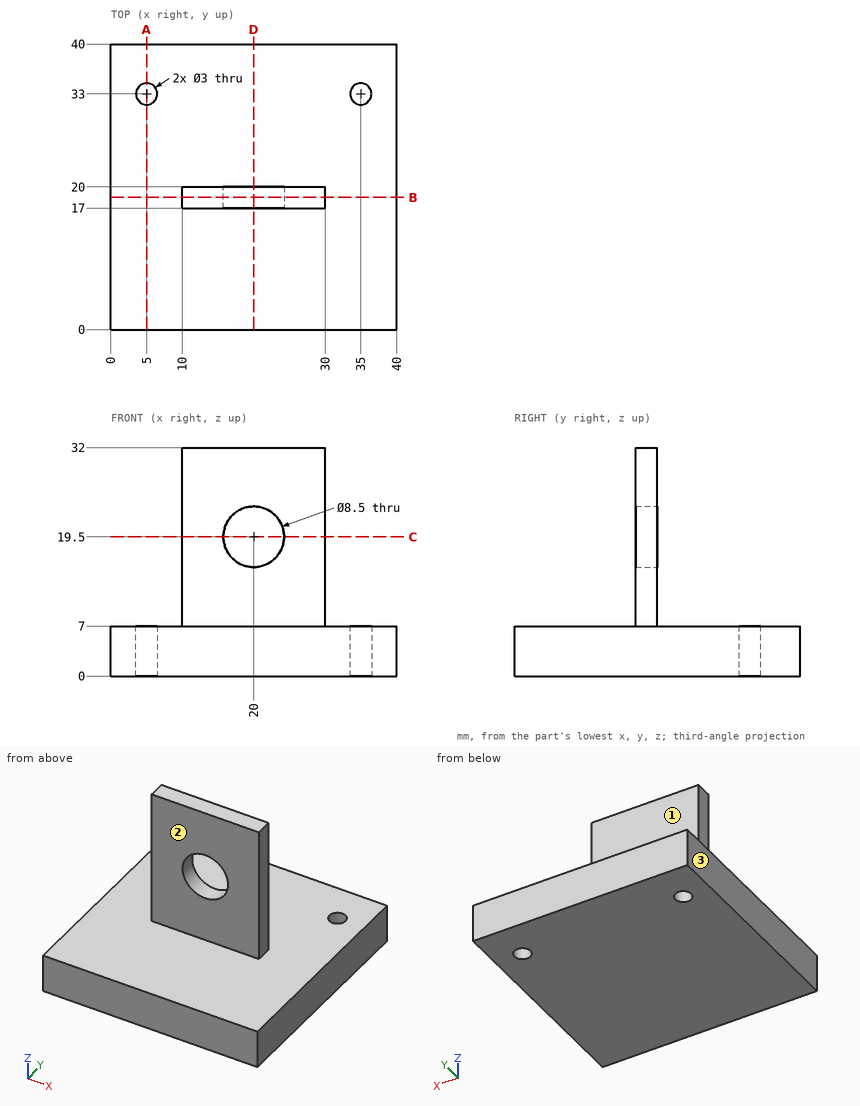
Geometry: see drawing. Coordinates: mm, zero at the bounding-box minimum. A direction names the side the tool comes from. Give positions to 0.01 mm unless a question says otherwise; leave off trailing zeros. Order: outer loops, then holes, each group sorted by start corner. A loop starts at its lowest first (then second) coordinate and runs counter-clockwise, first axis right, second up.
1. Cut plane B-B (y = 18.5). Return loops of the section in (x, z).
Computed:
outline: (0, 0) - (40, 0) - (40, 7) - (30, 7) - (30, 32) - (10, 32) - (10, 7) - (0, 7) - close; hole circle Ø8.5 at (20, 19.5)
2. Set-up query: the marked faces 1, 2 and 3. Return all of +Z, -Z, +X, -X, +Y, -Y with unobstructed straight access to the full face (end or side cutting, diameter ignored); none if empty.
Computed:
face 1: +Z, +X, -X, +Y
face 2: +Z, +X, -X, -Y
face 3: +Z, -Z, -X, +Y, -Y
3. Cut plane D-D (x = 20). Return loops of the section in (y, z), and give its area (4 significant figures).
Computed:
outline: (0, 0) - (40, 0) - (40, 7) - (20, 7) - (20, 15.25) - (17, 15.25) - (17, 7) - (0, 7) - close; (17, 23.75) - (20, 23.75) - (20, 32) - (17, 32) - close
area: 329.5 mm2
4. Cut plane C-C (z = 19.5). Return loops of the section in (x, y), and give its area (3 significant figures).
Computed:
outline: (10, 17) - (15.75, 17) - (15.75, 20) - (10, 20) - close; (24.25, 17) - (30, 17) - (30, 20) - (24.25, 20) - close
area: 34.5 mm2
5. Pin query (flat end, axial travel): pin 1 Ø10 at (x, z) = (23, 14) entering from -Y; pin 2 Ø4 at (x, y) = (35, 33) entering from +Z; pin 3 Ø6 at (x, z) = (14.5, 11) entering from +Y. Return the tip coordinate at first contact, or that it passes through.
Computed:
pin 1: stops at y = 17
pin 2: stops at z = 7
pin 3: stops at y = 20
6. Line query: probe 1 along Y at (x, z) = (5, 3.5); probe 2 along X at (y, z) = (18.2, 19.5); probe 3 along Y at (x, z) = (11, 9.5). Output: solid intervals per line, ascending.
Computed:
probe 1: y = 0 to 31.5, 34.5 to 40
probe 2: x = 10 to 15.75, 24.25 to 30
probe 3: y = 17 to 20
7. Cut plane A-A (x = 5). Return loops of the section in (y, z), and give its area (3 significant figures).
Computed:
outline: (0, 0) - (31.5, 0) - (31.5, 7) - (0, 7) - close; (34.5, 0) - (40, 0) - (40, 7) - (34.5, 7) - close
area: 259 mm2
